Answer from the drawing. Dimensions are ordinates in mm from the lowest x, y and z of the part. A direction names the side the tool comes from. Coordinates: 2 decimals unless noted, no trailing zeros. Order: outer loops, then holes, each group sorted by start corner. A loop starts at its lowest first (then second) coordinate and runs counter-clockwise, first axis right, second up. Notation, with made-up numbers: (19, 34.5) - (23, 34.5) arc R33 ccw to (23, 65.5) - close; hole circle Ø6 at (-3, 33). An arc over 180 degrees is marked (long way). Answer as a JSON object with one key per item and string values. Group by question number.
1) Find the intervals of material crossed by line 1 along X through (y, z) = (181.5, 174.5); line 2 along X through (y, z) = (61.5, 129); line 3 along Z through (x, y) = (348.5, 260.5) (1 decimal), in increasing order.
2) Section B-B (x = 351) is taken. Give the vertices of the cut face in (y, z) (1 decimal), plus the area to 3 significant figures.
3) Section C-C (z = 42) is taken. Give the vertices of the cut face in (x, y).
4) Each of these flat-tipped pins is pushed along its axis until it touches: P1, Ø4, axis at x = 225, z = 57.5, coming from the -Y side; P2, Ø20, axis at y = 235, z = 226.5, coming from the -X side; P3, Ø24, axis at x = 40, y = 96.5, coming from the +Z side. Where does it stop, or does it pass through?
5) Section D-D (y = 223.5) is taken. Give the vertices of the cut face in (x, z) (1 decimal), plus the area to 3 significant figures.
6) Section A-A (z = 152.5) is taken. Give the vertices of the cut face in (x, y).
7) The mould has two halves that part along X. Classify the marked faces 5, 6 and 7: released by +X, released by -X, zero draft, split by the parting line, or undercut.
8) A tool of negligible diameter and unlimited length cuts with its end or side. For the marked faces 1, 2, 3 and 4, from which of +Z, -Z, +X, -X, +Y, -Y can it reach the whole face along a straight path? Write none if from no direction.
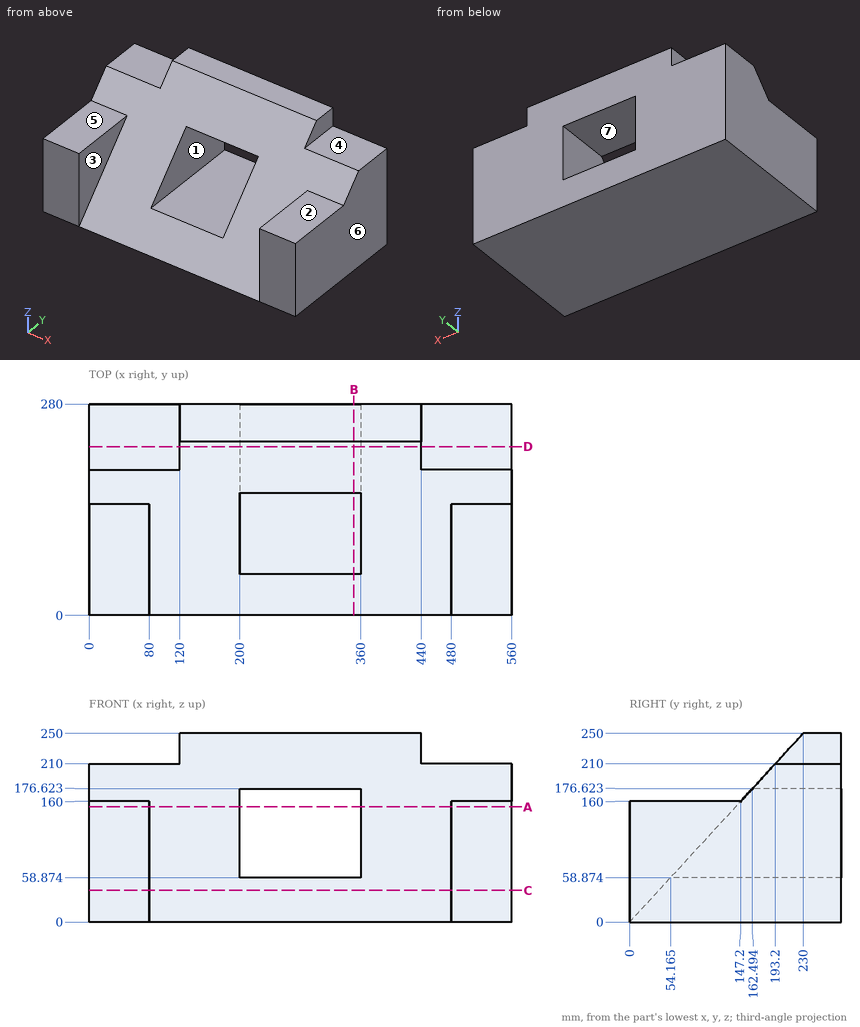
Report:
{
 "1": {"line 1": "x = 0 to 200, 360 to 560", "line 2": "x = 0 to 80, 480 to 560", "line 3": "z = 0 to 58.9, 176.6 to 250"},
 "2": {"outline": "(0, 0) - (280, 0) - (280, 58.9) - (54.2, 58.9) - close; (162.5, 176.6) - (280, 176.6) - (280, 250) - (230, 250) - close", "area": "21,000 mm²"},
 "3": {"outline": "(0, 0) - (80, 0) - (80, 38.64) - (480, 38.64) - (480, 0) - (560, 0) - (560, 280) - (0, 280) - close"},
 "4": {"P1": "stops at y = 51.06", "P2": "stops at x = 120", "P3": "stops at z = 160"},
 "5": {"outline": "(0, 0) - (560, 0) - (560, 210) - (440, 210) - (440, 242.9) - (120, 242.9) - (120, 210) - (0, 210) - close; hole (200, 58.9) - (360, 58.9) - (360, 176.6) - (200, 176.6) - close", "area": "109,000 mm²"},
 "6": {"outline": "(0, 0) - (80, 0) - (80, 140.3) - (200, 140.3) - (200, 280) - (0, 280) - close; (360, 140.3) - (480, 140.3) - (480, 0) - (560, 0) - (560, 280) - (360, 280) - close"},
 "7": {"face 5": "zero draft", "face 6": "released by +X", "face 7": "undercut"},
 "8": {"face 1": "+Y, -Y", "face 2": "+Z, +X, -X, -Y", "face 3": "+Z, -Y", "face 4": "+Z, +X, +Y, -Y"}
}
